For this review, take the finished solid that the model builds, in its own axes (mm). Round coordinates to 2 decimals unless told otherwise and drop trailing zeros. Loops run counter-clockwise (first coordinate to the right, second up) from the corner with the lowest first, then second, coordinate; pieces in that order, holes last. Notation, with made-up numbers: (68.25, 71.5) -> (112.25, 71.5) arc R24 cw to (112.25, 95.5) -> close; hole circle Ø8 at (-16, 39). An arc over 180 degrees is marked (long way). One line per question, with ' | ' between items. Start each with the question number.
1. Wall thickness on line 1 along Y through (x, z) = (-28.5, -2.5); line 2 along Z through (x, y) = (5, 21); line 3 along Z through (x, y) = (19, -5): over which ranges is each line inside the solid? List them lowest first.
2. Draft analysis for pull direction Y (two halves, no side actions). For faces 1 (the face through (-0.513, -18.607, 14.868)), 2 (the face through (-23.009, -8.771, 2.258)), 3 (the face through (-23.009, 8.771, 2.258)), 4 (the face through (-1, 0, -30.234)), state which applies: pulls with the +Y half, pulls with the -Y half, needs draft (parallel to the pull), parting line crosses it, or undercut.
3. Consider section B-B (z = 3.5). Write out the cut boundary in (x, y), and give its area (3 significant figures).
4. For pin 1 Ø10 at (x, y) = (8.5, 22.5) entering from +Z; pin 2 Ø1.5 at (x, y) = (-16, 3) entering from +Z; pin 3 Ø2 at (x, z) = (12, 13.5) entering from +Y, all flat-tipped, find the tip position at first contact; note any pin that passes through.
5. Consider section D-D (x = 14). Write out the cut boundary in (y, z), and give its area (3 significant figures).
6. Consider section A-A (x = -17). Write out the cut boundary in (y, z).
7. Consider section C-C (y = -13). Write out the cut boundary in (x, z).
```python
from build123d import *

# Parameters (mm, degrees)
F0_W     = 73.3171850443
F0_H     = 60.4678094387
F1_DEPTH = 30.8
F3_DEPTH = 61.601
F5_DEPTH = 73.3181850443


# Not quite as in the source:
# - a feature of the source that left no trace in its solid (it failed there, or was rolled back) is left out


with BuildPart() as f1:
    # F0 (on Front) → F1 (new body, symmetric)
    with BuildSketch(Plane.XZ):
        Rectangle(F0_W, F0_H)
    extrude(amount=F1_DEPTH, both=True)

    # F2 (on face) → F3 (cut, through all)
    with BuildSketch(Plane.XZ.offset(30.8)):
        Polygon((-36.6585925221, 30.2339047194), (-36.6585925221, 4.7981617972), (0, 30.2339047194), align=None)
        Polygon((36.6585925221, 30.2339047194), (0, 30.2339047194), (36.6585925221, 4.7981617972), align=None)
    extrude(amount=-F3_DEPTH, mode=Mode.SUBTRACT)

    # F4 (on face) → F5 (cut, through all)
    with BuildSketch(Plane(origin=(-36.6585925221, 0, 0), x_dir=(0, -1, 0), z_dir=(-1, 0, 0))):
        Polygon((0, 30.2339047194), (-30.8, 30.2339047194), (-30.8, 4.7981617972), align=None)
        Polygon((30.8, 30.2339047194), (0, 30.2339047194), (30.8, 4.7981617972), align=None)
    extrude(amount=-F5_DEPTH, mode=Mode.SUBTRACT)

    # F10: sweep along a path in F9
    with BuildLine(Plane(origin=(-9.9452522809, 6.8577617895, 6.0293064075), x_dir=(-0.4343419548, -0.8613999118, 0.2633196883), z_dir=(-0.7366055839, 0.5079273491, 0.4465669287))) as f10_path:
        Line((7.9611823679, -9.5022734797), (43.7169324882, -14.9015133699))
    # F6 (on Front) → F10 (sweep, cut)
    with BuildSketch(Plane.XZ):
        Polygon((-36.6585925221, 4.7981617972), (-36.6585925221, -30.2339047194), (0, 30.2339047194), align=None)
    sweep(path=f10_path.line, mode=Mode.SUBTRACT)

    # F11: F1 across plane


with BuildPart() as f1_1:
    add(f1.part)
    add(f1.part.mirror(Plane.XZ), mode=Mode.INTERSECT)


solid = f1_1.part
```
Answer block:
1) line 1: y = -30.8 to -12.55, 12.55 to 30.8 | line 2: z = -30.23 to 12.89 | line 3: z = -30.23 to 17.05
2) face 1: pulls with the -Y half | face 2: undercut | face 3: undercut | face 4: needs draft
3) outline: (-36.66, -30.8) -> (36.66, -30.8) -> (36.66, 30.8) -> (-36.66, 30.8) -> (-36.66, 29.66) -> (-16.21, 0) -> (-36.66, -29.66) -> close | area: 3,910 mm2
4) pin 1: stops at z = 15.78 | pin 2: stops at z = 8.76 | pin 3: stops at y = 21.47
5) outline: (-30.8, -30.23) -> (30.8, -30.23) -> (30.8, 4.8) -> (11.76, 20.52) -> (-11.76, 20.52) -> (-30.8, 4.8) -> close | area: 2,830 mm2
6) outline: (-30.8, -30.23) -> (30.8, -30.23) -> (30.8, 4.8) -> (14.28, 18.44) -> (0, 2.19) -> (-14.28, 18.44) -> (-30.8, 4.8) -> close
7) outline: (-36.66, -30.23) -> (36.66, -30.23) -> (36.66, 4.8) -> (15.47, 19.5) -> (-15.47, 19.5) -> (-36.66, -15.45) -> close
